Work out the finished part from the listing and answer in its coordinate system (mm). A direction names the side the tool comes from. Round coordinates to 2 decimals unless told otherwise and drop trailing zeros. Write each loop counter-clockwise with the first axis right and the second up, starting at its lowest first coordinate (ties: lowest second). Pieces come first, ordered by that corner, then holes. Notation, with made-up numbers: M 64.25,15.25 L 107.25,15.25 A19 ccw 107.25,25.25 Z; hole C -27.75,62.5 d1. An arc over 180 degrees is marked long. One line per item, written item: value. Start each with the question number.
Q1. Find section A-A (z = 0). Write down the section's boundary in (x, y).
Q2. A tool of negligible diameter and unlimited length cuts with its end or side. For faces 1 (the flat face through (2, 4.5, 0)), 2 (the flat face through (0.63, 3.76, 1.08)), 3 (the cylindrical face through (-1.5, -1.39, -0.07)), from which of +Z, -Z, +X, -X, +Y, -Y can it reach the whole face along a straight path? Write none if from no direction.
Q3. Find section C-C (y = 2.25). Write down the section's boundary in (x, z).
Q4. Given pin 1 Ø1 at (y, z) = (-1.5, 1) entering from -X; pin 2 Ø2 at (x, z) = (-0.5, 0) entering from +Y; pin 3 Ø1.5 at (y, z) = (-3.5, 1.5) entering from +X, each flat-ended and moving along its own axis, determine where each tip first touches the part or whether it passes through.
Q5. The mould has two halves that part along X. Classify faces 4 (the cylindrical face through (-0.596, 3.018, 2.685)), 5 (the flat face through (1.25, 4, 0)), 6 (the flat face through (0, -4.5, 0)): released by +X, released by -X, zero draft, split by the parting line, or undercut.
Q6. Find section B-B (y = -1.5). Write down the section's boundary in (x, z), and give its area (3 significant figures).
Q7. Consider probe 1 along Y at (x, z) = (-1.2, 2.1); probe 2 along Z at (x, y) = (-1.1, 4); probe 3 along Y at (x, z) = (-0.25, 0.2). Determine where each line is inside the solid, lowest interval first.
Autodesk Inventor part; units mm, degrees
ref_plane "YZ Plane" through (0, 0, 0) normal (1, 0, 0) x (0, 1, 0)
ref_plane "XZ Plane" through (0, 0, 0) normal (0, 1, 0) x (-1, 0, 0)
ref_plane "XY Plane" through (0, 0, 0) normal (0, 0, 1) x (1, 0, 0)
sketch "Sketch1" plane through (0, 0, 0) normal (0, 0, 1) x (1, 0, 0)
  line L0 (0, 4.5) -> (0, -4.5)
  line L1 (0, -4.5) -> (1.25, -4.5)
  line L2 (1.25, -4.5) -> (1.5, -4.25)
  line L3 (1.5, -4.25) -> (1.5, 1.4)
  line L4 (1.6, 1.5) -> (2.5, 1.5)
  line L5 (2.75, 1.75) -> (2.75, 4.25)
  line L6 (2.5, 4.5) -> (0, 4.5)
  arc A0 (1.6, 1.5) -> (1.5, 1.4) centre (1.6, 1.4) ccw
  line L7 (2.5, 4.5) -> (2.75, 4.25)
  line L8 (2.5, 1.5) -> (2.75, 1.75)
  point P0 (0, 0)
  point P1 (2.75, 1.5)
  point P2 (2.75, 4.5)
  point P3 (0, 0)
  dimension "d0" = 5.5
  dimension "d1" = 3
  dimension "d3" = 3
  dimension "d4" = 3.2
  dimension "d5" = 135
  dimension "d6" = 0.25
  dimension "d7" = 6
  dimension "d18" = 0.25
revolve "Revolution1" add sketch "Sketch1" angle 360 about axis through (0, 4.5, 0) along (0, -1, 0)
sketch "Sketch2" plane through (0, 4.5, 0) normal (0, 1, 0) x (1, 0, 0)
  line L0 (0, -1.4434) -> (-1.25, -0.7217)
  line L1 (-1.25, -0.7217) -> (-1.25, 0.7217)
  line L2 (-1.25, 0.7217) -> (0, 1.4434)
  line L3 (0, 1.4434) -> (1.25, 0.7217)
  line L4 (1.25, 0.7217) -> (1.25, -0.7217)
  line L5 (1.25, -0.7217) -> (0, -1.4434)
  point P0 (0, 0)
  point P1 (0, 0)
  dimension "d11" = 2.5
extrude "Extrusion1" cut sketch "Sketch2" against normal blind 1.5
thread "Thread1"
sketch "Sketch3" plane through (0, 0, 0) normal (1, 0, 0) x (0, 1, 0)
  line L0 (4.5, 1.4434) -> (4.5, 0.7217)
  line L1 (4.5, 1.4434) -> (4, 0.9434)
  line L2 (4, 0.9434) -> (4.5, 0.9434)
  line L3 (4.5, 0.9434) -> (4.5, 1.4434)
  line L4 (-0.8, 0) -> (4.8, 0)
  point P0 (0, 0)
  dimension "d16" = 0.5
revolve "Revolution2" cut sketch "Sketch3" angle 360 about axis through (0, -10, 0) along (0, 1, 0)
properties part number "Bolt_M3x0.35_6mm_SH" material "Stainless Steel"
The answers:
1. outline: M -2.75,1.75 L -2.5,1.5 L -1.6,1.5 A0.1 cw -1.5,1.4 L -1.5,-4.25 L -1.25,-4.5 L 1.25,-4.5 L 1.5,-4.25 L 1.5,1.4 A0.1 cw 1.6,1.5 L 2.5,1.5 L 2.75,1.75 L 2.75,4.25 L 2.5,4.5 L 1.44,4.5 L 1.25,4.31 L 1.25,3 L -1.25,3 L -1.25,4.31 L -1.44,4.5 L -2.5,4.5 L -2.75,4.25 Z
2. face 1: +Z, -Z, +X, -X, +Y
2. face 2: +Y
2. face 3: -Y
3. outline: C 0,0 d5.5
4. pin 1: x = -1.41
4. pin 2: y = 4.5
4. pin 3: x = 1.3
5. face 4: split by the parting line
5. face 5: undercut
5. face 6: zero draft
6. outline: C 0,0 d3
6. area: 7.07 mm2
7. probe 1: 1.5 to 4.5
7. probe 2: -2.52 to -0.81, 0.81 to 2.52
7. probe 3: -4.5 to 3
